from build123d import *

# Parameters (mm, degrees)
F1_DEPTH  = 12.7
F2_R      = 50.8
F3_DEPTH  = 99.06
F5_DEPTH  = 12.7
F6_R      = 25.4
F7_DEPTH  = 101.6
F8_R      = 38.1
F9_DEPTH  = 12.7
F10_R     = 22.429205
F11_DEPTH = 101.6
F12_R     = 6.592238
F13_DEPTH = 124.461
F14_R     = 5.08
F15_R     = 28.288722
F16_DEPTH = 124.461


with BuildPart() as f1:
    # F0 (on Top) → F1 (new body)
    with BuildSketch(Plane.XY):
        Polygon((-63.5, 63.5), (-63.5, 0), (-63.5, -63.5), (0, -63.5), (63.5, -63.5), (63.5, 0), (63.5, 63.5), (0, 63.5), align=None)
    extrude(amount=F1_DEPTH)

    # F2 (on face) → F3 (join)
    with BuildSketch(Plane.XY.offset(12.7)):
        Circle(F2_R)
    extrude(amount=F3_DEPTH)

    # F4 (on face) → F5 (join)
    with BuildSketch(Plane.XY.offset(111.76)):
        Polygon((-63.5, 63.5), (-63.5, 0), (-63.5, -63.5), (0, -63.5), (63.5, -63.5), (63.5, 0), (63.5, 63.5), (0, 63.5), align=None)
    extrude(amount=F5_DEPTH)

    # F6 (on Front) → F7 (join)
    with BuildSketch(Plane.XZ):
        with Locations((0, 59.307985)):
            Circle(F6_R)
    extrude(amount=F7_DEPTH)

    # F8 (on face) → F9 (join)
    with BuildSketch(Plane.XZ.offset(101.6)):
        with Locations((0, 59.307985)):
            Circle(F8_R)
    extrude(amount=F9_DEPTH)

    # F10 (on face) → F11 (cut)
    with BuildSketch(Plane.XZ.offset(114.3)):
        with Locations((0, 59.307985)):
            Circle(F10_R)
    extrude(amount=-F11_DEPTH, mode=Mode.SUBTRACT)

    # F12 (on face) → F13 (cut, through all)
    with BuildSketch(Plane.XY.offset(124.46)):
        with Locations((-51.887672, 50.463643)):
            Circle(F12_R)
        with Locations((51.887672, 50.463643)):
            Circle(F12_R)
        with Locations((51.887672, -50.463643)):
            Circle(F12_R)
        with Locations((-51.887672, -50.463643)):
            Circle(F12_R)
    extrude(amount=-F13_DEPTH, mode=Mode.SUBTRACT)

    # F14
    f14_edges = [f1.edges().sort_by_distance(p)[0] for p in [
        (63.5, -63.5, 118.11),
        (63.5, 63.5, 118.11),
        (63.5, 63.5, 6.35),
        (63.5, -63.5, 6.35),
        (-63.5, -63.5, 118.11),
        (-63.5, -63.5, 6.35),
        (-63.5, 63.5, 118.11),
        (-63.5, 63.5, 6.35),
    ]]
    fillet(f14_edges, radius=F14_R)

    # F15 (on face) → F16 (cut, through all)
    with BuildSketch(Plane.XY.offset(124.46)):
        Circle(F15_R)
    extrude(amount=-F16_DEPTH, mode=Mode.SUBTRACT)


solid = f1.part
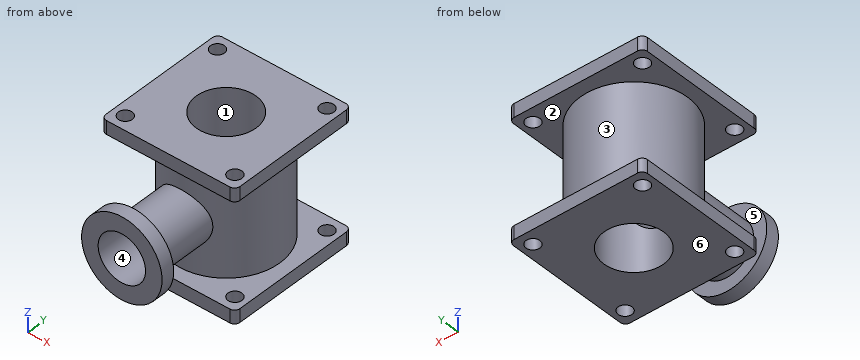
Source: CAD feature listing. Evaluate the final solid. Frame: model axes, mm. Face numbers are marked on the shaded views. A direction names the side the tool comes from. Round coordinates to 2 decimals unless told otherwise and drop trailing zeros. Write each loop counter-clockwise with the first axis right and the second up, starting at its lowest first coordinate (ties: lowest second). Pieces come first, ordered by that corner, then holes. Notation, with made-up numbers: (-27, 0.25) - (-6, 0.25) arc R24 ccw to (-6, 10.25) - close; hole circle Ø6 at (-9.75, 26). An arc over 180 degrees is marked (long way). Use CSV: the item, a comma, the result in double quotes. Start each with the question number.
(1) First-contact query: pin 1 Ø6.5 at (x, z) = (-12.5, 121) entering from -Y; pin 2 Ø5 at (y, z) = (33, 106) entering from -X (3 decimals); pin 3 Ø12 at (x, z) = (-19.5, 105.5) entering from +Y. Flat tips, straight axial feed; report the tip coordinate or a pass-through.
(2) Cut plane A-A, the plane y = 0. Return loops of the section in (x, z).
(3) Cut plane C-C, the plane z = 94.5. Return loops of the section in (x, y), and give its area (3 significant figures).
(4) Set-up query: the marked faces 5 and 6. Return all of +Z, -Z, +X, -X, +Y, -Y with unobstructed straight access to the full face (end or side cutting, diameter ignored); none if empty.
(5) Material intervals for probe 1 along Z at (x, y) = (0, -46); probe 2 along Z at (x, y) = (8, 54); probe 3 along Z at (x, y) = (-2, -54), sorted ascending. Write a range as [from, to].
(6) Cut plane D-D, the plane x = -55. Return loops of the section in (y, z), and give its area (3 significant figures).
(7) Mould query, pull axis X, two halves, no side actions, for the marked faces 1, 2, 3 and 4. Classes: pulls with the +X half, pulls with the -X half, needs draft (parallel to the pull), parting line crosses it, or undercut.
(8) Cut plane B-B, the plane x = 0. Return loops of the section in (y, z).
Geometry says:
1,pin 1,"y = -63.5"
1,pin 2,"x = -40.625"
1,pin 3,"y = 48.97"
2,outline,"(-63.5, 0) - (-28.29, 0) - (-28.29, 124.46) - (-63.5, 124.46) - (-63.5, 111.76) - (-50.8, 111.76) - (-50.8, 12.7) - (-63.5, 12.7) - close; (28.29, 0) - (63.5, 0) - (63.5, 12.7) - (50.8, 12.7) - (50.8, 111.76) - (63.5, 111.76) - (63.5, 124.46) - (28.29, 124.46) - close"
3,outline,"circle Ø101.6 at (0, 0); (-14.6, -114.3) - (14.6, -114.3) - (14.6, -101.6) - (-14.6, -101.6) - close; hole circle Ø56.58 at (0, 0)"
3,area,"5,960 mm²"
4,face 5,"none"
4,face 6,"-Z, +X, -X, +Y, -Y"
5,probe 1,"[0, 36.88], [81.74, 124.46]"
5,probe 2,"[0, 12.7], [111.76, 124.46]"
5,probe 3,"[0, 12.7], [33.99, 36.97], [81.65, 84.63], [111.76, 124.46]"
6,outline,"(-63.5, 0) - (-56.27, 0) - (-56.27, 12.7) - (-63.5, 12.7) - close; (-63.5, 111.76) - (-56.27, 111.76) - (-56.27, 124.46) - (-63.5, 124.46) - close; (-44.65, 0) - (44.65, 0) - (44.65, 12.7) - (-44.65, 12.7) - close; (-44.65, 111.76) - (44.65, 111.76) - (44.65, 124.46) - (-44.65, 124.46) - close; (56.27, 0) - (63.5, 0) - (63.5, 12.7) - (56.27, 12.7) - close; (56.27, 111.76) - (63.5, 111.76) - (63.5, 124.46) - (56.27, 124.46) - close"
6,area,"2,640 mm²"
7,face 1,"undercut"
7,face 2,"needs draft"
7,face 3,"parting line crosses it"
7,face 4,"undercut"
8,outline,"(-114.3, 21.21) - (-101.6, 21.21) - (-101.6, 33.91) - (-50.8, 33.91) - (-50.8, 12.7) - (-63.5, 12.7) - (-63.5, 0) - (-28.29, 0) - (-28.29, 36.88) - (-114.3, 36.88) - close; (-114.3, 81.74) - (-28.29, 81.74) - (-28.29, 124.46) - (-63.5, 124.46) - (-63.5, 111.76) - (-50.8, 111.76) - (-50.8, 84.71) - (-101.6, 84.71) - (-101.6, 97.41) - (-114.3, 97.41) - close; (28.29, 0) - (63.5, 0) - (63.5, 12.7) - (50.8, 12.7) - (50.8, 111.76) - (63.5, 111.76) - (63.5, 124.46) - (28.29, 124.46) - close"
